from build123d import *

# Parameters (mm, degrees)
SKETCH1_R                = 2.25
SKETCH1_R_2              = 12.6
SKETCH1_W                = 3
SKETCH1_H                = 4
SKETCH1_H_2              = 45
SKETCH1_W_2              = 9
SKETCH1_H_3              = 28
BOSS_EXTRUDE1_DEPTH      = 3
BOSS_EXTRUDE2_DEPTH      = 3
BOSS_EXTRUDE2_DEPTH_BACK = 7.3
SKETCH1_23_R             = 12.6
SKETCH1_23_R_2           = 9.6
BOSS_EXTRUDE3_DEPTH      = 3
BOSS_EXTRUDE3_DEPTH_BACK = 2.3
SKETCH1_24_R             = 9.6
SKETCH1_24_R_2           = 7
CUT_EXTRUDE1_DEPTH       = 110.735090103
CUT_EXTRUDE1_DEPTH_BACK  = 110.735090103
SKETCH2_R                = 7
SKETCH2_R_2              = 1.55
BOSS_EXTRUDE4_DEPTH      = 3
BOSS_EXTRUDE4_DEPTH_BACK = 5.25
SKETCH1_25_W             = 29.6
SKETCH1_25_H             = 8.3
SKETCH1_25_R             = 2.25


with BuildPart() as part:
    # Sketch1 → Boss-Extrude1 (new body)
    # profile 1 of 11: a face of its own
    with BuildSketch(Plane(origin=(0, 0, 0), x_dir=(1, 0, 0), z_dir=(0, 1, 0))):
        with BuildLine():
            Line((-27, -91.5), (-27, -97.5))
            ThreePointArc((-27, -97.5), (-22, -102.5), (-17, -97.5))
            Line((-17, -97.5), (-17, -91.5))
            Line((-17, -91.5), (-27, -91.5))
        make_face()
        Polygon((-19.834936491, -100), (-17.669872981, -96.25), (-19.834936491, -92.5), (-24.165063509, -92.5), (-26.330127019, -96.25), (-24.165063509, -100), align=None, mode=Mode.SUBTRACT)
    # profile 2 of 11: a face of its own
    with BuildSketch(Plane(origin=(0, 0, 0), x_dir=(1, 0, 0), z_dir=(0, 1, 0))):
        Polygon((-24.165063509, -100), (-19.834936491, -100), (-17.669872981, -96.25), (-19.834936491, -92.5), (-24.165063509, -92.5), (-26.330127019, -96.25), align=None)
        with Locations(Location((-22, -96.25, 0), (0, 0, 270))):
            Circle(SKETCH1_R, mode=Mode.SUBTRACT)
    # profile 3 of 11: a face of its own
    with BuildSketch(Plane(origin=(0, 0, 0), x_dir=(1, 0, 0), z_dir=(0, 1, 0))):
        Polygon((25.8, -8.6), (-27, -8.6), (-27, -42.5), (-24, -42.5), (-24, -87.5), (-14.76, -87.5), (-10, -79), (19, -79), (19, -51), (28, -51), align=None)
        with Locations(Location((0, -34, 0), (0, 0, 270))):
            Circle(SKETCH1_R_2, mode=Mode.SUBTRACT)
    # profile 4 of 11: a face of its own
    with BuildSketch(Plane(origin=(0, 0, 0), x_dir=(1, 0, 0), z_dir=(0, 1, 0))):
        Polygon((-14.76, -87.5), (-24, -87.5), (-24, -91.5), (-17, -91.5), align=None)
    # profile 5 of 11: a face of its own
    with BuildSketch(Plane(origin=(0, 0, 0), x_dir=(1, 0, 0), z_dir=(0, 1, 0))):
        with Locations((-25.5, -89.5)):
            Rectangle(SKETCH1_W, SKETCH1_H)
    # profile 6 of 11: a face of its own
    with BuildSketch(Plane(origin=(0, 0, 0), x_dir=(1, 0, 0), z_dir=(0, 1, 0))):
        with Locations((-25.5, -65)):
            Rectangle(SKETCH1_W, SKETCH1_H_2)
    # profile 7 of 11: a face of its own
    with BuildSketch(Plane(origin=(0, 0, 0), x_dir=(1, 0, 0), z_dir=(0, 1, 0))):
        with Locations((23.5, -65)):
            Rectangle(SKETCH1_W_2, SKETCH1_H_3)
    # profile 8 of 11: a face of its own
    with BuildSketch(Plane(origin=(0, 0, 0), x_dir=(1, 0, 0), z_dir=(0, 1, 0))):
        with BuildLine():
            Line((35, -51), (28, -51))
            Line((28, -51), (28, -79))
            Line((28, -79), (35, -79))
            ThreePointArc((35, -79), (37.474873734, -77.974873734), (38.5, -75.5))
            Line((38.5, -75.5), (38.5, -54.5))
            ThreePointArc((38.5, -54.5), (37.474873734, -52.025126266), (35, -51))
        make_face()
        Polygon((32.75, -78.330127019), (29, -76.165063509), (29, -71.834936491), (32.75, -69.669872981), (36.5, -71.834936491), (36.5, -76.165063509), align=None, mode=Mode.SUBTRACT)
        Polygon((36.5, -58.165063509), (32.75, -60.330127019), (29, -58.165063509), (29, -53.834936491), (32.75, -51.669872981), (36.5, -53.834936491), align=None, mode=Mode.SUBTRACT)
    # profile 9 of 11: a face of its own
    with BuildSketch(Plane(origin=(0, 0, 0), x_dir=(1, 0, 0), z_dir=(0, 1, 0))):
        Polygon((32.75, -69.669872981), (29, -71.834936491), (29, -76.165063509), (32.75, -78.330127019), (36.5, -76.165063509), (36.5, -71.834936491), align=None)
        with Locations(Location((32.75, -74, 0), (0, 0, 270))):
            Circle(SKETCH1_R, mode=Mode.SUBTRACT)
    # profile 10 of 11: a face of its own
    with BuildSketch(Plane(origin=(0, 0, 0), x_dir=(1, 0, 0), z_dir=(0, 1, 0))):
        Polygon((29, -53.834936491), (29, -58.165063509), (32.75, -60.330127019), (36.5, -58.165063509), (36.5, -53.834936491), (32.75, -51.669872981), align=None)
        with Locations(Location((32.75, -56, 0), (0, 0, 270))):
            Circle(SKETCH1_R, mode=Mode.SUBTRACT)
    # profile 11 of 11: a face of its own
    with BuildSketch(Plane(origin=(0, 0, 0), x_dir=(1, 0, 0), z_dir=(0, 1, 0))):
        Polygon((-27, -8.6), (-20.8, -4.6), (-14.8, -4.6), (14.8, -4.6), (20.8, -4.6), (25.8, -8.6), align=None)
    extrude(amount=BOSS_EXTRUDE1_DEPTH)

    # Sketch1_23 → Boss-Extrude2 (add, two sides: drawn at the far end of the back side and taken through both)
    with BuildSketch(Plane(origin=(0, 0, 0), x_dir=(1, 0, 0), z_dir=(0, 1, 0)).offset(-BOSS_EXTRUDE2_DEPTH_BACK)):
        with Locations(Location((0, -34, 0), (0, 0, 270))):
            Circle(SKETCH1_23_R)
        with Locations(Location((0, -34, 0), (0, 0, 270))):
            Circle(SKETCH1_23_R_2, mode=Mode.SUBTRACT)
    extrude(amount=BOSS_EXTRUDE2_DEPTH + BOSS_EXTRUDE2_DEPTH_BACK)

    # Sketch1_24 → Boss-Extrude3 (add, two sides: drawn at the far end of the back side and taken through both)
    with BuildSketch(Plane(origin=(0, 0, 0), x_dir=(1, 0, 0), z_dir=(0, 1, 0)).offset(-BOSS_EXTRUDE3_DEPTH_BACK)):
        with Locations(Location((0, -34, 0), (0, 0, 270))):
            Circle(SKETCH1_24_R)
        with Locations(Location((0, -34, 0), (0, 0, 270))):
            Circle(SKETCH1_24_R_2, mode=Mode.SUBTRACT)
    extrude(amount=BOSS_EXTRUDE3_DEPTH + BOSS_EXTRUDE3_DEPTH_BACK)

    # Sketch2 → Cut-Extrude1 (cut, two sides: drawn at the far end of the back side and taken through both)
    with BuildSketch(Plane(origin=(0, 0, 0), x_dir=(1, 0, 0), z_dir=(0, 1, 0)).offset(-CUT_EXTRUDE1_DEPTH_BACK)):
        with Locations(Location((0, -34, 0), (0, 0, 270))):
            Circle(SKETCH2_R)
        with Locations(Location((-8.5, -25.5, 0), (0, 0, 63.553985628))):
            Circle(SKETCH2_R_2)
        with Locations(Location((8.5, -25.5, 0), (0, 0, 116.446014372))):
            Circle(SKETCH2_R_2)
        with Locations(Location((8.5, -42.5, 0), (0, 0, 26.446014372))):
            Circle(SKETCH2_R_2)
        with Locations(Location((-8.5, -42.5, 0), (0, 0, 153.553985628))):
            Circle(SKETCH2_R_2)
    extrude(amount=CUT_EXTRUDE1_DEPTH + CUT_EXTRUDE1_DEPTH_BACK, mode=Mode.SUBTRACT)

    # Sketch1_25 → Boss-Extrude4 (add, two sides: drawn at the far end of the back side and taken through both)
    # profile 1 of 2: a face of its own
    with BuildSketch(Plane(origin=(0, 0, 0), x_dir=(1, 0, 0), z_dir=(0, 1, 0)).offset(-BOSS_EXTRUDE4_DEPTH_BACK)):
        Polygon((-27, -8.6), (-20.8, -4.6), (-14.8, -4.6), (14.8, -4.6), (20.8, -4.6), (25.8, -8.6), align=None)
    # profile 2 of 2: a face of its own
    with BuildSketch(Plane(origin=(0, 0, 0), x_dir=(1, 0, 0), z_dir=(0, 1, 0)).offset(-BOSS_EXTRUDE4_DEPTH_BACK)):
        with Locations((0, -0.45)):
            Rectangle(SKETCH1_25_W, SKETCH1_25_H)
        with Locations(Location((10, 0, 0), (0, 0, 270))):
            Circle(SKETCH1_25_R, mode=Mode.SUBTRACT)
        with Locations(Location((-10, 0, 0), (0, 0, 270))):
            Circle(SKETCH1_25_R, mode=Mode.SUBTRACT)
    extrude(amount=BOSS_EXTRUDE4_DEPTH + BOSS_EXTRUDE4_DEPTH_BACK)


solid = part.part
Build history of the part. All positions in model axes, mm. A direction names the side the tool comes from. Round coordinates to 2 decimals unless told otherwise and drop trailing zeros. Write each loop counter-clockwise with the first axis right and the second up, starting at its lowest first coordinate (ties: lowest second). Pieces come first, ordered by that corner, then holes. Notation, with made-up numbers: M -3.75,66.5 L 13.25,66.5 A30 cw 13.25,88.5 Z; hole C 17,72.25 d1. An arc over 180 degrees is marked long. Answer in a Markdown table with one row per item.
1. Flat gauge pins, fed straight in: P1, Ø3, axis at y = -1, z = 85, coming from the +X side; P2, Ø3.5, axis at x = -8.5, z = 25.5, coming from the +Y side; P3, Ø10, axis at x = 5.5, z = 0.5, coming from the -Y side; P4, Ø1.5, axis at x = 14, y = 1, coming from the +Z side. Where does each tip first touch, or does it go through?
Geometry check:
| item | result |
|---|---|
| P1 | x = -12.73 |
| P2 | y = 3 |
| P3 | y = -5.25 |
| P4 | z = 79 |
2. Probe L1, parallel to X at y = 2.1, z = 74; L2, parallel to Z at x = -1.5, y = -3.75; L3, parallel to X at y = -4.5, z = 33.5. List the from-to ranges inside material, lowest first. Write a range as [from, to].
Geometry check:
| item | result |
|---|---|
| L1 | [-27, 30.5], [35, 38.5] |
| L2 | [-3.7, 8.6], [21.49, 24.52], [43.48, 46.51] |
| L3 | [-12.59, -9.59], [9.59, 12.59] |
3. Saw through at B-B (x = -5.5). List the corners of the cut face in (y, z), and give its area (3 significant figures).
Geometry check:
| item | result |
|---|---|
| outline | M -7.3,22.66 L 0,22.66 L 0,8.6 L -5.25,8.6 L -5.25,-3.7 L 3,-3.7 L 3,29.67 L -2.3,29.67 L -2.3,26.13 L -7.3,26.13 Z; M -7.3,41.87 L -2.3,41.87 L -2.3,38.33 L 3,38.33 L 3,79 L 0,79 L 0,45.34 L -7.3,45.34 Z |
| area | 354 mm2 |
4. Mould opens along X. For faces 6 (the face through (-7.53, -1.08, 41.29)), 7 (the face through (0, -5.25, 4)), 8 (the face through (14.8, -1, 1)) say: +X half, -X half, draft (parallel to the pull), parting line (faces both ways), or undercut.
Geometry check:
| item | result |
|---|---|
| face 6 | undercut |
| face 7 | draft |
| face 8 | +X half |
5. Saw through at A-A (z = 56). List the corners of the cut face in (x, y), and give its area (3 significant figures).
Geometry check:
| item | result |
|---|---|
| outline | M -27,0 L 30.5,0 L 30.5,3 L -27,3 Z; M 35,0 L 38.5,0 L 38.5,3 L 35,3 Z |
| area | 183 mm2 |
6. Saw through at C-C (z = 0). List the corners of the cut face in (x, y).
Geometry check:
| item | result |
|---|---|
| outline | M -14.8,-5.25 L -12.25,-5.25 L -12.25,3 L -14.8,3 Z; M -7.75,-5.25 L 7.75,-5.25 L 7.75,3 L -7.75,3 Z; M 12.25,-5.25 L 14.8,-5.25 L 14.8,3 L 12.25,3 Z |
7. Which spindle directions (+Z, -Z, +X, -X, +Y, -Y) get a long thin tool onto all of the face, cutting with end or side? Do faces 1 (the face through (-14.8, -1, 1)), 2 (the face through (32, 1, 51)), 3 (the face through (-0.1, -3.7, 46.6)), 4 (the face through (-6, -2.3, 38)), 5 (the face through (-12.6, -3.7, 33.9)). Say none if no direction does.
Geometry check:
| item | result |
|---|---|
| face 1 | -Z, -X, +Y, -Y |
| face 2 | -Z, +X, +Y, -Y |
| face 3 | +Z, -Y |
| face 4 | -Y |
| face 5 | -X, -Y |
8. Saw through at D-D (y = 1.5). State how many separate pieces and enclosed holes the cut face has, and give its area (3 significant figures).
Geometry check:
| item | result |
|---|---|
| separate pieces | 1 |
| enclosed holes | 10 |
| area | 4,550 mm2 |
